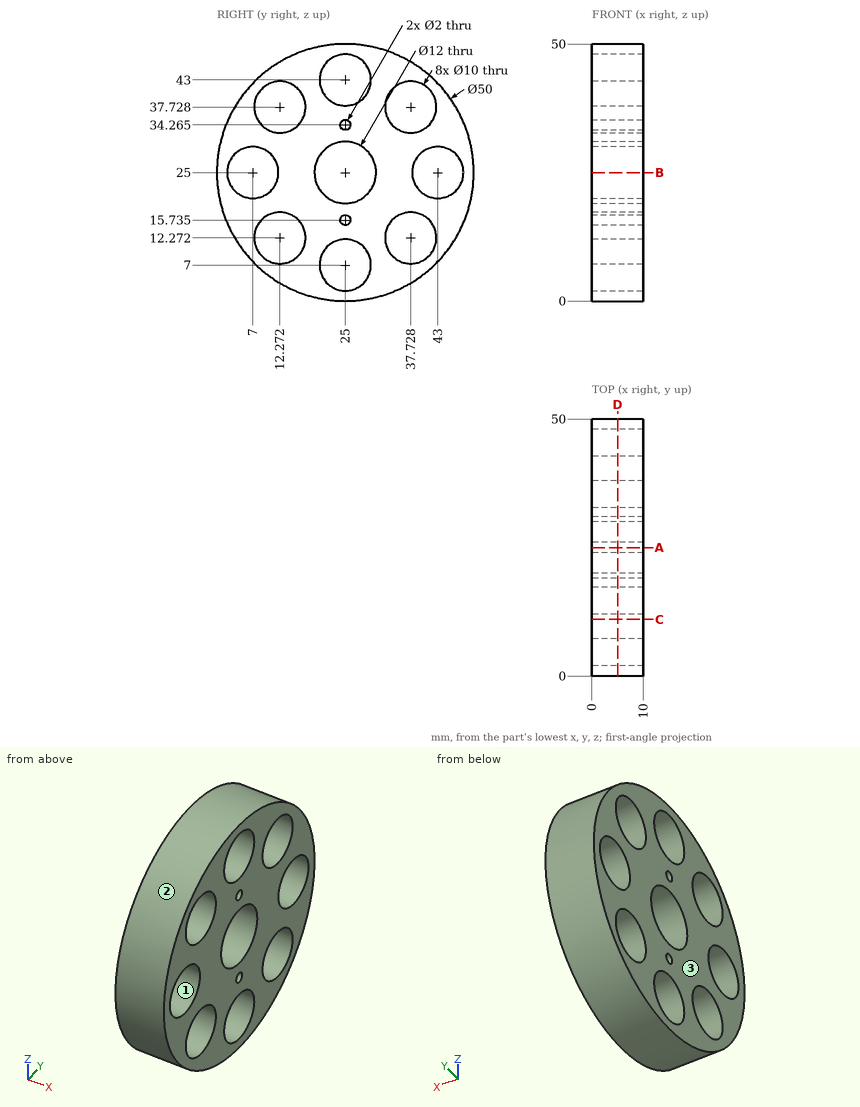
Geometry: see drawing. Coordinates: mm, zero at the bounding-box minimum. Coordinates: 2 decimals unless noted, no trailing zeros. Order: outer loops, then holes, each group sorted by start corner. A loop starts at its lowest first (then second) coordinate and runs counter-clockwise, first axis right, second up. Notation, with made-up numbers: M 87.5,87 L 121.5,87 A25 cw 121.5,109 Z; hole C 7.25,-21 d3. An arc over 180 degrees is marked long. Answer in a Markdown table with one row per item. Add a question column.
Q1. Section query C-C on y = 11. Return the cut outline in (x, z).
Q2. Mould query, pull axis Z, two halves, no side actions, for the marked faces 1, 2 and 3. Classes: released by +Z, released by -Z, zero draft, split by the parting line, or undercut.
Q3. Section query D-D on x = 5. Count the separate pieces of the cut face and the enclosed holes in it, and give its area (3 significant figures).
Q4. Section query B-B on z = 25. Return the cut outline in (x, y), and give its area (3 significant figures).
Q5. Line query: L1, parallel to Y at x = 2.75, z = 25; L2, parallel to Y at x = 6, z = 10.5 (1 decimal); L3, parallel to Z at x = 3.25, y = 9. Output: solid intervals per line, ascending.
Q6. Section query A-A on y = 25. Return the cut outline in (x, z) (3 decimals), and give its area (3 significant figures).
Q7. Contact query for flat-ended pins moving along their axis: P1, Ø1.5, axis at x = 8.5, y = 30, coming from the +Z side; P2, Ø4, axis at x = 8, z = 28, coming from the -Y side; P3, Ø1, axis at y = 40.5, z = 24.5, coming from the -X side; P4, Ø1, axis at x = 1.5, z = 30, coming from the +Y side. Output: stop coordinate, or through.
Completed:
| question | item | result |
|---|---|---|
| 1 | outline | M 0,4.29 L 10,4.29 L 10,7.44 L 0,7.44 Z; M 0,17.11 L 10,17.11 L 10,22 L 0,22 Z; M 0,28 L 10,28 L 10,32.89 L 0,32.89 Z; M 0,42.56 L 10,42.56 L 10,45.71 L 0,45.71 Z |
| 2 | face 1 | undercut |
| 2 | face 2 | split by the parting line |
| 2 | face 3 | zero draft |
| 3 | separate pieces | 1 |
| 3 | enclosed holes | 11 |
| 3 | area | 1,220 mm2 |
| 4 | outline | M 0,0 L 10,0 L 10,2 L 0,2 Z; M 0,12 L 10,12 L 10,19 L 0,19 Z; M 0,31 L 10,31 L 10,38 L 0,38 Z; M 0,48 L 10,48 L 10,50 L 0,50 Z |
| 4 | area | 180 mm2 |
| 5 | L1 | y = 0 to 2, 12 to 19, 31 to 38, 48 to 50 |
| 5 | L2 | y = 4.6 to 7.6, 16.9 to 21.4, 28.6 to 33.1, 42.4 to 45.4 |
| 5 | L3 | z = 5.79 to 8.49, 16.05 to 20.42, 29.58 to 33.95, 41.51 to 44.21 |
| 6 | outline | M 0,0 L 10,0 L 10,2 L 0,2 Z; M 0,12 L 10,12 L 10,14.735 L 0,14.735 Z; M 0,16.735 L 10,16.735 L 10,19 L 0,19 Z; M 0,31 L 10,31 L 10,33.265 L 0,33.265 Z; M 0,35.265 L 10,35.265 L 10,38 L 0,38 Z; M 0,48 L 10,48 L 10,50 L 0,50 Z |
| 6 | area | 140 mm2 |
| 7 | P1 | stops at z = 49.64 |
| 7 | P2 | stops at y = 0.02 |
| 7 | P3 | passes through |
| 7 | P4 | stops at y = 49.59 |
